The model under review builds one solid part; all positions refer to its coordinate system, in mm. A direction names the side the tool comes from. Coordinates: 2 decimals unless noted, no trailing zeros. Order: outer loops, then holes, each group sorted by start corner. A loop starts at its lowest first (then second) coordinate and runs counter-clockwise, first axis right, second up.
```python
from build123d import *

# Parameters (mm, degrees)
F1_DEPTH = 114.3
F2_R     = 5.08
F3_R     = 3.17499
F4_R     = 1.397


# Not quite as in the source:
# - a fillet or chamfer is up to 0.001 mm smaller than in the source, because OpenCascade refuses the exact size


with BuildPart() as f1:
    # F0 (on Front) → F1 (new body, symmetric)
    with BuildSketch(Plane.XZ):
        Polygon((76.2, 0), (0, 0), (0, -76.2), (6.35, -76.2), (6.35, -6.35), (76.2, -6.35), align=None)
    extrude(amount=F1_DEPTH, both=True)

    # F2
    f2_edges = [f1.edges().sort_by_distance(p)[0] for p in [
        (6.35, 0, -6.35),
    ]]
    fillet(f2_edges, radius=F2_R)

    # F3 (radius 3.175 in the source; OpenCascade refuses exactly that, so slightly less here)
    f3_edges = [f1.edges().sort_by_distance(p)[0] for p in [
        (76.2, 0, -6.35),
        (76.2, 0, 0),
        (0, 0, -76.2),
        (6.35, 0, -76.2),
    ]]
    fillet(f3_edges, radius=F3_R)

    # F4
    f4_edges = [f1.edges().sort_by_distance(p)[0] for p in [
        (0, 0, 0),
    ]]
    fillet(f4_edges, radius=F4_R)


solid = f1.part
```
(1) We need section C-C, the plane x = 24.5. Write out the cut boundary in (y, z), and give its area (3 significant figures).
A:
outline: (-114.3, -6.35) - (114.3, -6.35) - (114.3, 0) - (-114.3, 0) - close
area: 1,450 mm2
(2) Wall thickness on probe 1 along Z at (x, y) = (17, -61.5); probe 2 along X at (y, z) = (32, -13.5); probe 3 along Z at (x, y) = (5, -85): over which ranges is each line inside the solid? List them lowest first.
A:
probe 1: z = -6.35 to 0
probe 2: x = 0 to 6.35
probe 3: z = -75.62 to 0
(3) We need section B-B, the plane z = -54. Write out the cut boundary in (x, y).
A:
outline: (0, -114.3) - (6.35, -114.3) - (6.35, 114.3) - (0, 114.3) - close
(4) For pin 1 Ø6 at (x, y) = (10.5, 60.5) entering from -Z; pin 2 Ø2 at (y, z) = (29, -8.5) entering from +X; pin 3 Ø3 at (x, y) = (22, -64.5) entering from -Z, all flat-tipped, find the tip position at first contact; note any pin that passes through.
A:
pin 1: stops at z = -8.21
pin 2: stops at x = 8.21
pin 3: stops at z = -6.35
(5) Machinability: for faces 1 (the face through (42, -2, -6.35)), 2 (the face through (4, 114.3, -21)), which of the approach directions +Z, -Z, +X, -X, +Y, -Y give a long, thin tool a straight path to every point of the face, cutting with its end or side? Answer none if there is none.
A:
face 1: -Z, +X, +Y, -Y
face 2: +Z, -Z, +X, -X, +Y
